```python
from build123d import *

# Parameters (mm, degrees)
SCHIZZO1_W                     = 64.6
SCHIZZO1_H                     = 20
ESTRUSIONE_ESTRUSIONE1_DEPTH   = 8.2
SCHIZZO2_W                     = 8.2
SCHIZZO2_H                     = 20
ESTRUSIONE_ESTRUSIONE2_DEPTH   = 27.8
SCHIZZO3_W                     = 8.2
SCHIZZO3_H                     = 20
ESTRUSIONE_ESTRUSIONE3_DEPTH   = 27.8
SCHIZZO4_W                     = 8.2
SCHIZZO4_H                     = 20
ESTRUSIONE_ESTRUSIONE4_DEPTH   = 8.2
SCHIZZO5_W                     = 36
SCHIZZO5_H                     = 20
ESTRUSIONE_ESTRUSIONE5_DEPTH   = 8.2
SCHIZZO6_W                     = 48.2
SCHIZZO6_H                     = 19.6
TAGLIO_ESTRUSIONE1_DEPTH       = 77.610443152
F_4_0_4_DIAMETER_HOLE2_D       = 4
F_4_0_4_DIAMETER_HOLE2_DEPTH   = 8.2
SCHIZZO11_R                    = 16
ESTRUSIONE_ESTRUSIONE6_DEPTH   = 8.2
RACCORDO1_R                    = 10
F_22_0_22_DIAMETER_HOLE1_D     = 22
F_22_0_22_DIAMETER_HOLE1_DEPTH = 10
F_22_0_22_DIAMETER_HOLE1_TIP   = 6.609466809
RACCORDO3_R                    = 6
SCHIZZO15_W                    = 8.2
SCHIZZO15_H                    = 36
ESTRUSIONE_ESTRUSIONE7_DEPTH   = 3.5
SCHIZZO16_W                    = 8.2
SCHIZZO16_H                    = 36
ESTRUSIONE_ESTRUSIONE8_DEPTH   = 3.5
SCHIZZO17_W                    = 36
SCHIZZO17_H                    = 6
ESTRUSIONE_ESTRUSIONE9_DEPTH   = 11
RACCORDO6_R                    = 2
SCHIZZO23_R                    = 11
ESTRUSIONE_ESTRUSIONE10_DEPTH  = 2.2
ESTRUSIONE_ESTRUSIONE11_DEPTH  = 10
F_4_0_4_DIAMETER_HOLE1_D       = 4


with BuildPart() as part:
    # Schizzo1 → Estrusione-Estrusione1 (new body)
    with BuildSketch(Plane.XY):
        with Locations((32.3, 10)):
            Rectangle(SCHIZZO1_W, SCHIZZO1_H)
    extrude(amount=ESTRUSIONE_ESTRUSIONE1_DEPTH)

    # Schizzo2 → Estrusione-Estrusione2 (add)
    with BuildSketch(Plane.XY.offset(8.2)):
        with Locations((4.1, 10)):
            Rectangle(SCHIZZO2_W, SCHIZZO2_H)
    extrude(amount=ESTRUSIONE_ESTRUSIONE2_DEPTH)

    # Schizzo3 → Estrusione-Estrusione3 (add)
    with BuildSketch(Plane.XY.offset(8.2)):
        with Locations((60.5, 10)):
            Rectangle(SCHIZZO3_W, SCHIZZO3_H)
    extrude(amount=ESTRUSIONE_ESTRUSIONE3_DEPTH)

    # Schizzo4 → Estrusione-Estrusione4 (add)
    with BuildSketch(Plane.ZY.offset(-56.4)):
        with Locations((31.9, 10)):
            Rectangle(SCHIZZO4_W, SCHIZZO4_H)
    extrude(amount=ESTRUSIONE_ESTRUSIONE4_DEPTH)

    # Schizzo5 → Estrusione-Estrusione5 (add)
    with BuildSketch(Plane.ZY):
        with Locations((18, 10)):
            Rectangle(SCHIZZO5_W, SCHIZZO5_H)
    extrude(amount=ESTRUSIONE_ESTRUSIONE5_DEPTH)

    # Schizzo6 → Taglio-Estrusione1 (cut, through all)
    with BuildSketch(Plane.XZ):
        with Locations((24.1, 18)):
            Rectangle(SCHIZZO6_W, SCHIZZO6_H)
    extrude(amount=-TAGLIO_ESTRUSIONE1_DEPTH, mode=Mode.SUBTRACT)

    # Ø4.0 (4) Diameter Hole2
    with Locations(Plane.XY.offset(36)):
        with Locations((52.95, 5), (3.45, 5), (3.45, 15), (52.95, 15)):
            Hole(F_4_0_4_DIAMETER_HOLE2_D / 2, depth=F_4_0_4_DIAMETER_HOLE2_DEPTH)

    # Schizzo11 → Estrusione-Estrusione6 (add)
    with BuildSketch(Plane(origin=(0, 0, 0), x_dir=(-1, 0, 0), z_dir=(0, 0, -1))):
        with Locations((-38.3, 10)):
            Circle(SCHIZZO11_R)
    extrude(amount=-ESTRUSIONE_ESTRUSIONE6_DEPTH)

    # Raccordo1
    raccordo1_edges = [part.edges().sort_by_distance(p)[0] for p in [
        (50.789995997, 0, 4.1),
        (50.789995997, 20, 4.1),
        (25.810004003, 0, 4.1),
        (25.810004003, 20, 4.1),
    ]]
    fillet(raccordo1_edges, radius=RACCORDO1_R)

    # Ø22.0 (22) Diameter Hole1
    with Locations(Plane(origin=(0, 0, 0), x_dir=(-1, 0, 0), z_dir=(0, 0, -1))):
        with Locations((-38.3, 10)):
            Hole(F_22_0_22_DIAMETER_HOLE1_D / 2, depth=F_22_0_22_DIAMETER_HOLE1_DEPTH)
            with Locations((0, 0, -(F_22_0_22_DIAMETER_HOLE1_DEPTH + F_22_0_22_DIAMETER_HOLE1_TIP / 2))):  # 118° drill point
                Cone(0, F_22_0_22_DIAMETER_HOLE1_D / 2, F_22_0_22_DIAMETER_HOLE1_TIP, mode=Mode.SUBTRACT)

    # Raccordo3
    raccordo3_edges = [part.edges().sort_by_distance(p)[0] for p in [
        (64.6, 10, 36),
        (64.6, 10, 0),
    ]]
    fillet(raccordo3_edges, radius=RACCORDO3_R)

    # Schizzo15 → Estrusione-Estrusione7 (add)
    with BuildSketch(Plane.XZ):
        with Locations((-4.1, 18)):
            Rectangle(SCHIZZO15_W, SCHIZZO15_H)
    extrude(amount=ESTRUSIONE_ESTRUSIONE7_DEPTH)

    # Schizzo16 → Estrusione-Estrusione8 (add)
    with BuildSketch(Plane(origin=(0, 20, 0), x_dir=(1, 0, 0), z_dir=(0, 1, 0))):
        with Locations((-4.1, -18)):
            Rectangle(SCHIZZO16_W, SCHIZZO16_H)
    extrude(amount=ESTRUSIONE_ESTRUSIONE8_DEPTH)

    # Schizzo17 → Estrusione-Estrusione9 (add)
    with BuildSketch(Plane.ZY.offset(8.2)):
        with Locations((18, 20.5)):
            Rectangle(SCHIZZO17_W, SCHIZZO17_H)
        with Locations((18, -0.5)):
            Rectangle(SCHIZZO17_W, SCHIZZO17_H)
    extrude(amount=ESTRUSIONE_ESTRUSIONE9_DEPTH)

    # Raccordo6
    raccordo6_edges = [part.edges().sort_by_distance(p)[0] for p in [
        (0, -3.5, 18),
        (0, 23.5, 18),
    ]]
    fillet(raccordo6_edges, radius=RACCORDO6_R)

    # Schizzo23 → Estrusione-Estrusione10 (add)
    with BuildSketch(Plane.XY.offset(8.2)):
        with Locations(Location((38.3, 10, 0), (0, 0, 180))):
            Circle(SCHIZZO23_R)
    extrude(amount=-ESTRUSIONE_ESTRUSIONE10_DEPTH)

    # Schizzo24 → Estrusione-Estrusione11 (add)
    with BuildSketch(Plane.XY.offset(36)):
        with BuildLine():
            Line((-2, 23.5), (-19.2, 23.5))
            Line((-19.2, 23.5), (-19.2, 17.5))
            Line((-19.2, 17.5), (-8.2, 17.5))
            Line((-8.2, 17.5), (-8.2, 2.5))
            Line((-8.2, 2.5), (-19.2, 2.5))
            Line((-19.2, 2.5), (-19.2, -3.5))
            Line((-19.2, -3.5), (-2, -3.5))
            ThreePointArc((-2, -3.5), (-0.585786438, -2.914213562), (0, -1.5))
            Line((0, -1.5), (0, 21.5))
            ThreePointArc((0, 21.5), (-0.585786438, 22.914213562), (-2, 23.5))
        make_face()
    extrude(amount=ESTRUSIONE_ESTRUSIONE11_DEPTH)

    # Ø4.0 (4) Diameter Hole1 (through all)
    with Locations(Plane(origin=(0, -3.5, 0), x_dir=(-1, 0, 0), z_dir=(0, -1, 0))):
        with Locations((13.7, -37.1), (13.7, -9.1)):
            Hole(F_4_0_4_DIAMETER_HOLE1_D / 2)


solid = part.part
```
Model file for the job. Use its own axes, mm. A direction names the side the tool comes from. Coordinates: 2 decimals unless noted, no trailing zeros. Loops run counter-clockwise (first coordinate to the right, second up) from the corner with the lowest first, then second, coordinate; pieces in that order, holes last. Notation, with made-up numbers: (-38.75, 83) - (-17.75, 83) arc R17 cw to (-17.75, 109) - close; hole circle Ø4 at (56.25, 0.25). An arc over 180 degrees is marked (long way). Answer as a JSON object with one key per item and string values. Group by question number.
(1) Cut at D-D (x = 3.45). Give the cut face in (y, z), then the cut area to 3 significant figures.
(2) Flat gauge pins, fed straight in: pin 1 (10 mm diameter, centred on x = 25.5, z = 8.5, fed in from +Y); pin 2 (8.5 mm diameter, centred on x = -12.5, z = 31.5, fed in from -Y); pin 3 (4 mm diameter, centred on x = 3.5, z = 33.5, fed in from +Y). Where does each tip first touch, or does it go through?
(3) Cut at C-C (z = 9.1). Give the cut face in (x, y).
(4) Probe line 1 along Y through (x, z) = (52.95, 30.5); line 2 along Z through (x, y) = (-13.7, 19.6); line 3 along Z through (x, y) = (0.5, 10). List the from-to ranges inside material, lowest first.
(5) Tool access for faces 1 (the face through (3.71, 16.983, 31.843)), 2 (the face through (52, 10, 27.8)), 3 (the face through (-11, -3.5, 23)), 4 (the face through (53, 10, 36)): list every direction of +Z, -Z, +X, -X, +Y, -Y with a clear straight run to the whole face (end or side of a thin tool).
(6) Cut at A-A (z = 25). Give the cut face in (x, y).
(7) Cut at B-B (x = -13.7). Give the cut face in (y, z).
(8) Two-plate mould, pull along Z, no slides. Class faces 5 (the face through (62.889, 10.14, 34.196)), 6 (the face through (11, 0, 4)), 7 (the face through (-14.134, 20.542, 11.052)): released by +Z, released by -Z, zero draft, split by the parting line, or undercut.
Geometry says:
{
 "1": {"outline": "(0, 0) - (20, 0) - (20, 8.2) - (0, 8.2) - close; (0, 27.8) - (3, 27.8) - (3, 36) - (0, 36) - close; (7, 27.8) - (13, 27.8) - (13, 36) - (7, 36) - close; (17, 27.8) - (20, 27.8) - (20, 36) - (17, 36) - close", "area": "262 mm^2"},
 "2": {"pin 1": "stops at y = 23.96", "pin 2": "stops at y = -3.5", "pin 3": "stops at y = 20"},
 "3": {"outline": "(-19.2, -3.5) - (-15.7, -3.5) - (-15.7, 2.5) - (-19.2, 2.5) - close; (-19.2, 17.5) - (-15.7, 17.5) - (-15.7, 23.5) - (-19.2, 23.5) - close; (-11.7, -3.5) - (-2, -3.5) arc R2 ccw to (0, -1.5) - (0, 21.5) arc R2 ccw to (-2, 23.5) - (-11.7, 23.5) - (-11.7, 17.5) - (-8.2, 17.5) - (-8.2, 2.5) - (-11.7, 2.5) - close; (56.4, 0) - (64.6, 0) - (64.6, 20) - (56.4, 20) - close"},
 "4": {"line 1": "y = 0 to 3, 7 to 13, 17 to 20", "line 2": "z = 0 to 7.1, 11.1 to 35.1, 39.1 to 46", "line 3": "z = 0 to 8.2, 27.8 to 36"},
 "5": {"face 1": "+Z", "face 2": "+Y, -Y", "face 3": "+Z, -Z, -X, -Y", "face 4": "+Z, +X, +Y, -Y"},
 "6": {"outline": "(-19.2, -3.5) - (-2, -3.5) arc R2 ccw to (0, -1.5) - (0, 21.5) arc R2 ccw to (-2, 23.5) - (-19.2, 23.5) - (-19.2, 17.5) - (-8.2, 17.5) - (-8.2, 2.5) - (-19.2, 2.5) - close; (56.4, 0) - (64.6, 0) - (64.6, 20) - (56.4, 20) - close"},
 "7": {"outline": "(-3.5, 0) - (2.5, 0) - (2.5, 7.1) - (-3.5, 7.1) - close; (-3.5, 11.1) - (2.5, 11.1) - (2.5, 35.1) - (-3.5, 35.1) - close; (-3.5, 39.1) - (2.5, 39.1) - (2.5, 46) - (-3.5, 46) - close; (17.5, 0) - (23.5, 0) - (23.5, 7.1) - (17.5, 7.1) - close; (17.5, 11.1) - (23.5, 11.1) - (23.5, 35.1) - (17.5, 35.1) - close; (17.5, 39.1) - (23.5, 39.1) - (23.5, 46) - (17.5, 46) - close"},
 "8": {"face 5": "released by +Z", "face 6": "zero draft", "face 7": "undercut"}
}
